Source: CAD feature listing. Evaluate the final solid. Frame: model axes, mm. Coordinates: 2 decimals unless noted, no trailing zeros. Loops run counter-clockwise (first coordinate to the right, second up) from the corner with the lowest first, then second, coordinate; pieces in that order, holes last.
```python
from build123d import *

# Parameters (mm, degrees)
BOSS_EXTRUDE1_DEPTH    = 304.8
F_10_CLEARANCE_HOLE1_D = 5.1054


with BuildPart() as part:
    # Sketch1 → Boss-Extrude1 (new body)
    with BuildSketch(Plane.XY):
        with BuildLine():
            Line((-1.143, -8.256814656), (-1.143, 12.7))
            Line((-1.143, 12.7), (1.143, 12.7))
            Line((1.143, 12.7), (1.143, -12.7))
            ThreePointArc((1.143, -12.7), (-9.173985791, -15.198384078), (-1.143, -8.256814656))
        make_face()
    extrude(amount=BOSS_EXTRUDE1_DEPTH)

    # #10 Clearance Hole1 (through all)
    with Locations(Plane.ZY.offset(1.143)):
        with Locations((9.525, 0), (295.275, 0)):
            Hole(F_10_CLEARANCE_HOLE1_D / 2)


solid = part.part
```
Q1. First-contact query: pin 1 Ø6.5 at (y, z) = (0, 165) entering from -X; pin 2 Ø3 at (y, z) = (-8, 232.5) entering from -X; pin 3 Ø5 at (x, z) = (-8.5, 158) entering from -Y. Flat tips, straight axial feed; report the tip coordinate or a pass-through.
Q2. Section query C-C on x = -3.25. Return the cut outline in (y, z).
Q3. Material intervals for line 1 along X through (y, z) = (4, 219); line 2 along Y through (x, z) = (-4.25, 92.5); line 3 along X through (y, z) = (-8, 254), sorted ascending.
Q4. Section query A-A on y = 0. Return the cut outline in (x, z).
Q5. Draft query along Z for faces 1 (the flat face through (-3, -9, 304.8)), 2 (the cylindrical face through (0, 0.8, 7.1)), 3 (the flat face through (-3, -9, 0)). Return one class per face: released by +Z, released by -Z, zero draft, split by the parting line, or undercut.
Q6. Section query B-B on z = 105.5. Return the cut outline in (x, y).
Resolved:
1. pin 1: stops at x = -1.14
1. pin 2: stops at x = -8.74
1. pin 3: stops at y = -17.9
2. outline: (-18.06, 0) - (-7.34, 0) - (-7.34, 304.8) - (-18.06, 304.8) - close
3. line 1: x = -1.14 to 1.14
3. line 2: y = -18.16 to -7.24
3. line 3: x = -7.1 to -1.54, -1.14 to 1.14
4. outline: (-1.14, 0) - (1.14, 0) - (1.14, 6.97) - (-1.14, 6.97) - close; (-1.14, 12.08) - (1.14, 12.08) - (1.14, 292.72) - (-1.14, 292.72) - close; (-1.14, 297.83) - (1.14, 297.83) - (1.14, 304.8) - (-1.14, 304.8) - close
5. face 1: released by +Z
5. face 2: undercut
5. face 3: released by -Z
6. outline: (-1.14, -8.26) arc R5.46 ccw (long way) to (1.14, -12.7) - (1.14, 12.7) - (-1.14, 12.7) - close
